CAD build for the part. Positions are in the model's coordinates, mm. A direction names the side the tool comes from. Coordinates: 2 decimals unless noted, no trailing zeros. Order: outer loops, then holes, each group sorted by start corner. A loop starts at its lowest first (then second) coordinate and runs counter-clockwise, first axis right, second up. Notation, with made-up numbers: (47.5, 73.5) - (62.5, 73.5) arc R24 cw to (62.5, 102.5) - close; hole circle Ø8 at (26.25, 21). An arc over 180 degrees is marked (long way). Return JSON: item names as keys, results as strings.
from build123d import *

# Parameters (mm, degrees)
SKETCH_1_W      = 40
SKETCH_1_H      = 39
EXTRUDE_1_DEPTH = 10
SKETCH_2_R      = 4.432676277
EXTRUDE_4_DEPTH = 1
SKETCH_3_R      = 3.469401761
EXTRUDE_5_DEPTH = 1
SKETCH_5_R      = 2.620946211
EXTRUDE_6_DEPTH = 3
SKETCH_6_W      = 10
SKETCH_6_H      = 5.416587347
EXTRUDE_7_DEPTH = 10
SKETCH_7_W      = 10
SKETCH_7_H      = 5.249064027
EXTRUDE_8_DEPTH = 10


with BuildPart() as part:
    # 草图1 → 凸台-拉伸1 (new body)
    with BuildSketch(Plane.XY):
        with Locations((-12.52596939, -9.298515699)):
            Rectangle(SKETCH_1_W, SKETCH_1_H)
    extrude(amount=EXTRUDE_1_DEPTH)

    # 草图2 → 凸台-拉伸4 (add)
    with BuildSketch(Plane(origin=(0, 10.201484301, 0), x_dir=(1, 0, 0), z_dir=(0, 1, 0))):
        with Locations(Location((-26.216270459, -5.306111922, 0), (0, 0, 90))):
            Circle(SKETCH_2_R)
    extrude(amount=EXTRUDE_4_DEPTH)

    # 草图3 → 凸台-拉伸5 (add)
    with BuildSketch(Plane(origin=(0, 11.201484301, 0), x_dir=(1, 0, 0), z_dir=(0, 1, 0))):
        with Locations(Location((-26.216270459, -5.306111922, 0), (0, 0, 270))):
            Circle(SKETCH_3_R)
    extrude(amount=EXTRUDE_5_DEPTH)

    # 草图5 → 凸台-拉伸6 (add)
    with BuildSketch(Plane(origin=(0, 12.201484301, 0), x_dir=(1, 0, 0), z_dir=(0, 1, 0))):
        with Locations(Location((-26.216270459, -5.306111922, 0), (0, 0, 270))):
            Circle(SKETCH_5_R)
    extrude(amount=EXTRUDE_6_DEPTH)

    # 草图6 → 凸台-拉伸7 (add)
    with BuildSketch(Plane.ZY.offset(32.52596939)):
        with Locations((5, 1.493888641)):
            Rectangle(SKETCH_6_W, SKETCH_6_H)
    extrude(amount=EXTRUDE_7_DEPTH)

    # 草图7 → 凸台-拉伸8 (add)
    with BuildSketch(Plane(origin=(7.47403061, 0, 0), x_dir=(0, 0, -1), z_dir=(1, 0, 0))):
        with Locations((-5, 2.080220262)):
            Rectangle(SKETCH_7_W, SKETCH_7_H)
    extrude(amount=EXTRUDE_8_DEPTH)


solid = part.part
Item 1: Band-saw the part on D-D, the plane x = -25.5. List the corners of the cut face in (y, z).
Findings below:
{"outline": "(-28.8, 0) - (10.2, 0) - (10.2, 0.93) - (11.2, 0.93) - (11.2, 1.91) - (12.2, 1.91) - (12.2, 2.78) - (15.2, 2.78) - (15.2, 7.83) - (12.2, 7.83) - (12.2, 8.7) - (11.2, 8.7) - (11.2, 9.68) - (10.2, 9.68) - (10.2, 10) - (-28.8, 10) - close"}
Item 2: Drop flat-ended pins along their axis: P1, Ø4, axis at y = 8.5, z = 8, coming from the -X side; P2, Ø3, axis at x = 14.5, z = 3.5, coming from the -Y side; P3, Ø1.5, axis at x = -2, z = 8, coming from the +Y side; P4, Ø1, axis at x = -35, y = -24, coming from the -Z side. Give the stop position or say it passes through.
Findings below:
{"P1": "stops at x = -32.53", "P2": "stops at y = -0.54", "P3": "stops at y = 10.2", "P4": "passes through"}
Item 3: Wall check: L1, parallel to Y at x = -14, z = 5.75; L2, parallel to X at y = 5, z = 3.75; L3, parallel to Y at x = 11.5, z = 3. Give the ranges that are in metal, low to high. Write a range as [from, to].
Findings below:
{"L1": "y = [-28.8, 10.2]", "L2": "x = [-32.53, 7.47]", "L3": "y = [-0.54, 4.7]"}
Item 4: Band-saw the part on A-A, the plane x = 9. List the corners of the cut face in (y, z).
Findings below:
{"outline": "(-0.54, 0) - (4.7, 0) - (4.7, 10) - (-0.54, 10) - close"}
Item 5: Band-saw the part on C-C, the plane y = -15.5. List the corners of the cut face in (x, z), then the cut area to 3 significant figures.
Findings below:
{"outline": "(-32.53, 0) - (7.47, 0) - (7.47, 10) - (-32.53, 10) - close", "area": "400 mm²"}
Item 6: Which spindle directions (+Z, -Z, +X, -X, +Y, -Y) get a long thin tool onto all of the face, cutting with end or side? Do faces 1 (the flat face through (-32.526, -15, 5)), 2 (the flat face through (7.474, -15, 5)), 3 (the cylindrical face through (-29.603, 11.694, 4.554)). Say none if no direction does.
Findings below:
{"face 1": "+Z, -Z, -X, -Y", "face 2": "+Z, -Z, +X, -Y", "face 3": "+Y"}
Item 7: Band-saw the part on B-B, the plane z = 5.5. List the corners of the cut face in (x, y).
Findings below:
{"outline": "(-42.53, -1.21) - (-32.53, -1.21) - (-32.53, -28.8) - (7.47, -28.8) - (7.47, -0.54) - (17.47, -0.54) - (17.47, 4.7) - (7.47, 4.7) - (7.47, 10.2) - (-21.79, 10.2) - (-21.79, 11.2) - (-22.75, 11.2) - (-22.75, 12.2) - (-23.6, 12.2) - (-23.6, 15.2) - (-28.83, 15.2) - (-28.83, 12.2) - (-29.68, 12.2) - (-29.68, 11.2) - (-30.64, 11.2) - (-30.64, 10.2) - (-32.53, 10.2) - (-32.53, 4.2) - (-42.53, 4.2) - close"}
